Autodesk Inventor part; units mm, degrees
ref_plane "YZ Plane" through (0, 0, 0) normal (1, 0, 0) x (0, 1, 0)
ref_plane "XZ Plane" through (0, 0, 0) normal (0, 1, 0) x (-1, 0, 0)
ref_plane "XY Plane" through (0, 0, 0) normal (0, 0, 1) x (1, 0, 0)
sketch "Sketch1" plane through (0, 0, 0) normal (0, 0, 1) x (1, 0, 0)
  circle A0 centre (0, 0) radius 1.5
  circle A1 centre (0, 0) radius 4.75
  dimension "d0" = 3
  dimension "d1" = 9.5
extrude "Extrusion1" add sketch "Sketch1" along normal blind 3
sketch "Sketch2" plane through (0, 0, 3) normal (0, 0, 1) x (1, 0, 0)
  circle A0 centre (0, 0) radius 4.75
  line L0 (4.5069, 1.5) -> (5.0069, 1.5)
  line L1 (5.0069, 1.5) -> (5.0069, -1.5)
  line L2 (5.0069, -1.5) -> (4.5069, -1.5)
  line L3 (4.5069, -1.5) -> (4.5069, 1.5)
  point P0 (4.5069, 0)
  dimension "d4" = 3
  dimension "d5" = 0.5
extrude "Extrusion2" add sketch "Sketch2" against normal blind 3 contours A0 L0 L1 L2
sketch "Sketch4" plane through (5.0069, -1.5, 3) normal (1, 0, 0) x (0, 0, -1)
  line L0 (-1.5, 3.5) -> (4.5, 3.5)
  line L1 (4.5, 3.5) -> (4.5, -0.5)
  line L2 (4.5, -0.5) -> (-1.5, -0.5)
  line L3 (-1.5, -0.5) -> (-1.5, 3.5)
  line L4 (0, 3) -> (3, 3)
  line L5 (0, 0) -> (0, 3)
  point P0 (3, 1.5)
  point P1 (1.5, 3)
  point P2 (1.5, 3.5)
  point P3 (0, 1.5)
  point P4 (-1.5, 1.5)
  dimension "d9" = 6
  dimension "d10" = 4
extrude "Extrusion3" add sketch "Sketch4" along normal blind 4
fillet "Fillet1" radius 1 4 edges at (7.0069, 2, 4.5) (7.0069, -2, 4.5) (7.0069, -2, -1.5) (7.0069, 2, -1.5)
sketch "Sketch6" plane through (9.0069, -1.5, 3) normal (1, 0, 0) x (0, 0, -1)
  circle A0 centre (1.5, 1.5) radius 1.5
  line L0 (3.5, 3.5) -> (-0.5, 3.5)
  line L1 (-1.5, 2.5) -> (-1.5, 0.5)
  point P0 (3, 1.5)
  point P1 (-1.5, 1.5)
  point P2 (1.5, 3.5)
  dimension "d14" = 3
extrude "Extrusion4" cut sketch "Sketch6" against normal blind 3
properties part number "Arm7" material "ABS Plastic"
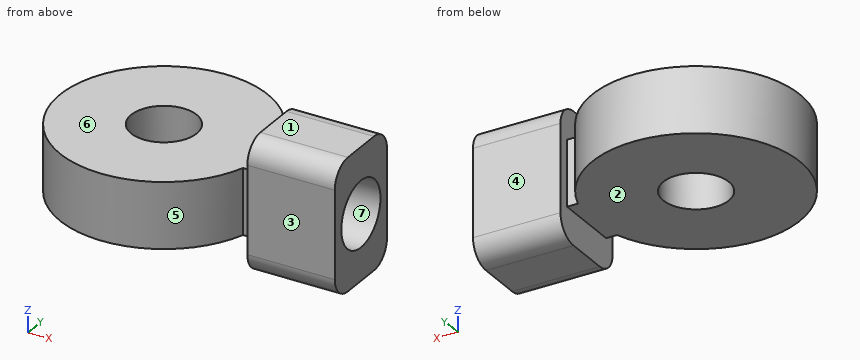
Build history of the part. All positions in model axes, mm. Face numbers are marked on the shaded views. A direction names the side the tool comes from. Round coordinates to 2 decimals unless told otherwise and drop trailing zeros. Write each loop counter-clockwise with the first axis right and the second up, starting at its lowest first coordinate (ties: lowest second). Pieces come first, ordered by that corner, then holes. Notation, with made-up numbers: M 19.5,-36 L 36.5,-36 A5 cw 36.5,-32 Z; hole C -5.75,-34 d8. An arc over 180 degrees is marked long. Answer in a Markdown table with one row per item.
1. Saw through at B-B (y = 0). List the corners of the cut face in (x, z), and give its area (3 significant figures).
Geometry check:
| item | result |
|---|---|
| outline | M -4.75,0 L -1.5,0 L -1.5,3 L -4.75,3 Z; M 1.5,0 L 5.01,0 L 5.01,-1.5 L 9.01,-1.5 L 9.01,0 L 6.01,0 L 6.01,3 L 9.01,3 L 9.01,4.5 L 5.01,4.5 L 5.01,3 L 1.5,3 Z |
| area | 35.3 mm2 |
2. Mould opens along Y. For the marked faces 5, 6 and 7 say: +Y half, -Y half, draft (parallel to the pull), parting line (faces both ways), or undercut.
Geometry check:
| item | result |
|---|---|
| face 5 | parting line |
| face 6 | draft |
| face 7 | undercut |
3. Saw through at A-A (x = 6.25). List the corners of the cut face in (y, z), and give its area (3 significant figures).
Geometry check:
| item | result |
|---|---|
| outline | M -2,-0.5 A1 ccw -1,-1.5 L 1,-1.5 A1 ccw 2,-0.5 L 2,3.5 A1 ccw 1,4.5 L -1,4.5 A1 ccw -2,3.5 Z; hole C 0,1.5 d3 |
| area | 16.1 mm2 |
4. Which spindle directions (+Z, -Z, +X, -X, +Y, -Y) get a long thin tool onto all of the face, cutting with end or side? Do the marked faces 1, 2, 3 and 4. Say none if no direction does.
Geometry check:
| item | result |
|---|---|
| face 1 | +Z, +X, -X, +Y, -Y |
| face 2 | -Z, -X, +Y, -Y |
| face 3 | +Z, -Z, +X, -Y |
| face 4 | +Z, -Z, +X, +Y |
5. Saw through at C-C (z = 1.15). List the corners of the cut face in (x, y).
Geometry check:
| item | result |
|---|---|
| outline | M 4.51,-1.5 L 5.01,-1.5 L 5.01,-2 L 9.01,-2 L 9.01,-1.46 L 6.01,-1.46 L 6.01,1.46 L 9.01,1.46 L 9.01,2 L 5.01,2 L 5.01,1.5 L 4.51,1.5 A4.75 ccw long Z; hole C 0,0 d3 |
6. Flat gauge pins, fed straight in: P1, Ø5, axis at x = 5, y = 3, coming from the -Z side; P2, Ø1.2, axis at x = 7, z = 1.5, coming from the -Y side; P3, Ø4, axis at x = 0, y = 0, coming from the +Z side; P4, Ø1.5, axis at y = 1, z = 2.5, coming from the -X side. Where does each tip first touch, or does it go through?
Geometry check:
| item | result |
|---|---|
| P1 | z = -1.5 |
| P2 | y = -2 |
| P3 | z = 3 |
| P4 | x = -4.74 |
7. Probe L1, parallel to Y at x = 7.95, z = 1.5; L2, parallel to Y at x = 0, z = 1.7; L3, parallel to Z at x = 2.75, y = 2.75. List the from-to ranges inside material, lowest first. Write a range as [from, to].
Geometry check:
| item | result |
|---|---|
| L1 | [-2, -1.5], [1.5, 2] |
| L2 | [-4.75, -1.5], [1.5, 4.75] |
| L3 | [0, 3] |
8. Saw through at D-D (x = 0). List the corners of the cut face in (y, z), and give its area (3 significant figures).
Geometry check:
| item | result |
|---|---|
| outline | M -4.75,0 L -1.5,0 L -1.5,3 L -4.75,3 Z; M 1.5,0 L 4.75,0 L 4.75,3 L 1.5,3 Z |
| area | 19.5 mm2 |
